Geometry: final body of the model. Coordinates: model frame, mm. Coordinates: 2 decimals unless noted, no trailing zeros. Order: outer loops, then holes, each group sorted by start corner. A loop starts at its lowest first (then second) coordinate and runs counter-clockwise, first axis right, second up. Notation, with made-up numbers: M 43.25,-37 L 93.25,-37 A27 cw 93.25,-19 Z; hole C 61,-0.75 d8. An arc over 180 degrees is marked long. Write item = value, one per line. Start each with the question number.
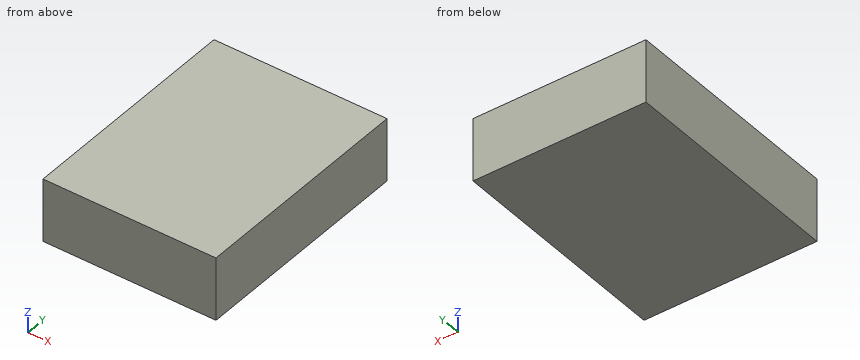
```python
from build123d import *

# Parameters (mm, degrees)
F0_W     = 265
F0_H     = 95
F1_DEPTH = 350
F2_T     = -1.5
F3_W     = 265
F3_H     = 350
F4_DEPTH = 1.5


with BuildPart() as f1:
    # F0 (on Front) → F1 (new body)
    with BuildSketch(Plane.XZ):
        with Locations((132.5, 47.5)):
            Rectangle(F0_W, F0_H)
    extrude(amount=-F1_DEPTH)

    # F2
    f2_openings = [f1.faces().sort_by_distance(p)[0] for p in [
        (132.5, 175, 95),
    ]]
    offset(amount=F2_T, openings=f2_openings)

    # F3 (on face) → F4 (join)
    with BuildSketch(Plane.XY.offset(95)):
        with Locations((132.5, 175)):
            Rectangle(F3_W, F3_H)
    extrude(amount=F4_DEPTH)


solid = f1.part
```
Item 1: Material intervals for probe 1 along Y at (x, z) = (104, 69.5); probe 2 along X at (y, z) = (269, 7); probe 3 along Z at (x, y) = (191, 316), sorted ascending. Write a range as [from, to].
Item 2: Section query A-A on z = 83.5. Output: boundary loops of the cut face in (x, y).
Item 3: Section query B-B on y = 137. Output: boundary loops of the cut face in (x, z).
Ans:
q1.probe_1 = [0, 1.5], [348.5, 350]
q1.probe_2 = [0, 1.5], [263.5, 265]
q1.probe_3 = [0, 1.5], [95, 96.5]
q2.outline = M 0,0 L 265,0 L 265,350 L 0,350 Z; hole M 1.5,1.5 L 263.5,1.5 L 263.5,348.5 L 1.5,348.5 Z
q3.outline = M 0,0 L 265,0 L 265,96.5 L 0,96.5 Z; hole M 1.5,1.5 L 263.5,1.5 L 263.5,95 L 1.5,95 Z
